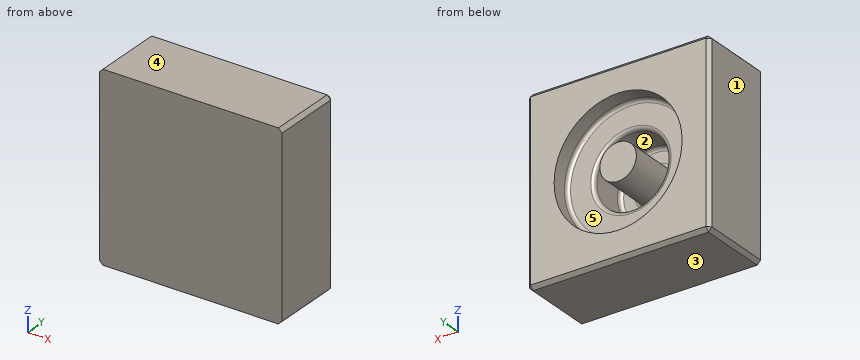
from build123d import *

# Parameters (mm, degrees)
SKETCH1_W           = 63.5
SKETCH1_H           = 63.5
BOSS_EXTRUDE1_DEPTH = 25.4
SKETCH2_R           = 22.225
CUT_EXTRUDE1_DEPTH  = 6.35
SKETCH3_R           = 12.7
CUT_EXTRUDE2_DEPTH  = 12.7
SKETCH4_R           = 6.35
BOSS_EXTRUDE2_DEPTH = 19.05
FILLET1_R           = 1.27
CHAMFER1_SIZE       = 1.27


with BuildPart() as part:
    # Sketch1 → Boss-Extrude1 (new body)
    with BuildSketch(Plane(origin=(0, 0, 0), x_dir=(1, 0, 0), z_dir=(0, 1, 0))):
        Rectangle(SKETCH1_W, SKETCH1_H)
    extrude(amount=BOSS_EXTRUDE1_DEPTH)

    # Sketch2 → Cut-Extrude1 (cut)
    with BuildSketch(Plane(origin=(0, 25.4, 0), x_dir=(1, 0, 0), z_dir=(0, 1, 0))):
        with Locations(Location((0, 0, 0), (0, 0, 270))):
            Circle(SKETCH2_R)
    extrude(amount=-CUT_EXTRUDE1_DEPTH, mode=Mode.SUBTRACT)

    # Sketch3 → Cut-Extrude2 (cut)
    with BuildSketch(Plane(origin=(0, 19.05, 0), x_dir=(1, 0, 0), z_dir=(0, 1, 0))):
        with Locations(Location((0, 0, 0), (0, 0, 270))):
            Circle(SKETCH3_R)
    extrude(amount=-CUT_EXTRUDE2_DEPTH, mode=Mode.SUBTRACT)

    # Sketch4 → Boss-Extrude2 (add)
    with BuildSketch(Plane(origin=(0, 6.35, 0), x_dir=(1, 0, 0), z_dir=(0, 1, 0))):
        with Locations(Location((0, 0, 0), (0, 0, 270))):
            Circle(SKETCH4_R)
    extrude(amount=BOSS_EXTRUDE2_DEPTH)

    # Fillet1
    fillet1_edges = [part.edges().sort_by_distance(p)[0] for p in [
        (0, 19.05, -22.225),
        (0, 6.35, -12.7),
        (0, 19.05, -12.7),
        (0, 6.35, -6.35),
    ]]
    fillet(fillet1_edges, radius=FILLET1_R)

    # Chamfer1
    chamfer1_edges = [part.edges().sort_by_distance(p)[0] for p in [
        (-31.75, 25.4, 0),
        (0, 25.4, 31.75),
        (31.75, 25.4, 0),
        (0, 25.4, -31.75),
        (31.75, 12.7, 31.75),
        (-31.75, 12.7, 31.75),
        (-31.75, 12.7, -31.75),
        (31.75, 12.7, -31.75),
    ]]
    chamfer(chamfer1_edges, length=CHAMFER1_SIZE)


solid = part.part
Can you work these out from the model? Positions are in its coordinate system, mm. Face numbers are marked on the shaded views. A direction names the side the tool comes from. Coordinates: 2 decimals unless noted, no trailing zeros. Write each loop counter-clockwise with the first axis right and the second up, starting at its lowest first coordinate (ties: lowest second). Pieces come first, ordered by that corner, then holes. Notation, with made-up numbers: (4.5, 26.5) - (47.5, 26.5) arc R14 cw to (47.5, 38.5) - close; hole circle Ø1 at (1, 31). An arc over 180 degrees is marked (long way). Return JSON: item names as keys, results as strings. Group by question number.
Item 1: Please list where these lines run through material, in increasing order: probe 1 along X at (y, z) = (13, 0); probe 2 along Z at (x, y) = (2, 10.5); probe 3 along Y at (x, z) = (0, 10).
Item 2: If we section it at A-A (y = 16.75): Write out the boundary of the cut face in (x, z), then the cut area to 3 significant figures.
Item 3: Which directions (+Z, -Z, +X, -X, +Y, -Y) give clear straight access to the entire face, cutting with the end or side of a thin tool? Please do the marked faces 4 and 5.
Item 4: We'd pull the mould along Z, two halves only. Please class the marked faces 1, 2 and 3: pulls with the +Z half, pulls with the -Z half, needs draft (parallel to the pull), parting line crosses it, or undercut.
Item 5: If we section it at C-C (z = 0): Write out the boundary of the cut face in (x, y) (3 decimals), then the cut area to 3 significant figures.
Item 6: I'm going to push flat-ended pins straight in: pin 1 Ø1 at (x, z) = (18, 8) entering from +Y; pin 2 Ø3 at (x, z) = (2.5, -8.5) entering from +Y. Where does each tip first touch, or does it pass through?
Item 7: If we section it at B-B (x = 0): Write out the boundary of the cut face in (y, z) (3 decimals), then the cut area to 3 significant figures.
Return value:
{
 "1": {"probe 1": "x = -31.75 to -12.7, -6.35 to 6.35, 12.7 to 31.75", "probe 2": "z = -31.75 to -12.54, -6.03 to 6.03, 12.54 to 31.75", "probe 3": "y = 0 to 6.35"},
 "2": {"outline": "(-31.75, -30.48) - (-30.48, -31.75) - (30.48, -31.75) - (31.75, -30.48) - (31.75, 30.48) - (30.48, 31.75) - (-30.48, 31.75) - (-31.75, 30.48) - close; circle Ø12.7 at (0, 0); hole circle Ø25.4 at (0, 0)", "area": "3,650 mm^2"},
 "3": {"face 4": "+Z, +X, -X, +Y, -Y", "face 5": "+Y"},
 "4": {"face 1": "needs draft", "face 2": "undercut", "face 3": "pulls with the -Z half"},
 "5": {"outline": "(-31.75, 0) - (31.75, 0) - (31.75, 24.13) - (30.48, 25.4) - (22.225, 25.4) - (22.225, 20.32) arc R1.27 cw to (20.955, 19.05) - (13.97, 19.05) arc R1.27 ccw to (12.7, 17.78) - (12.7, 7.62) arc R1.27 cw to (11.43, 6.35) - (7.62, 6.35) arc R1.27 cw to (6.35, 7.62) - (6.35, 25.4) - (-6.35, 25.4) - (-6.35, 7.62) arc R1.27 cw to (-7.62, 6.35) - (-11.43, 6.35) arc R1.27 cw to (-12.7, 7.62) - (-12.7, 17.78) arc R1.27 ccw to (-13.97, 19.05) - (-20.955, 19.05) arc R1.27 cw to (-22.225, 20.32) - (-22.225, 25.4) - (-30.48, 25.4) - (-31.75, 24.13) - close", "area": "1,250 mm^2"},
 "6": {"pin 1": "stops at y = 19.05", "pin 2": "stops at y = 6.38"},
 "7": {"outline": "(0, -31.75) - (24.13, -31.75) - (25.4, -30.48) - (25.4, -22.225) - (20.32, -22.225) arc R1.27 cw to (19.05, -20.955) - (19.05, -13.97) arc R1.27 ccw to (17.78, -12.7) - (7.62, -12.7) arc R1.27 cw to (6.35, -11.43) - (6.35, -7.62) arc R1.27 cw to (7.62, -6.35) - (25.4, -6.35) - (25.4, 6.35) - (7.62, 6.35) arc R1.27 cw to (6.35, 7.62) - (6.35, 11.43) arc R1.27 cw to (7.62, 12.7) - (17.78, 12.7) arc R1.27 ccw to (19.05, 13.97) - (19.05, 20.955) arc R1.27 cw to (20.32, 22.225) - (25.4, 22.225) - (25.4, 30.48) - (24.13, 31.75) - (0, 31.75) - close", "area": "1,250 mm^2"}
}
